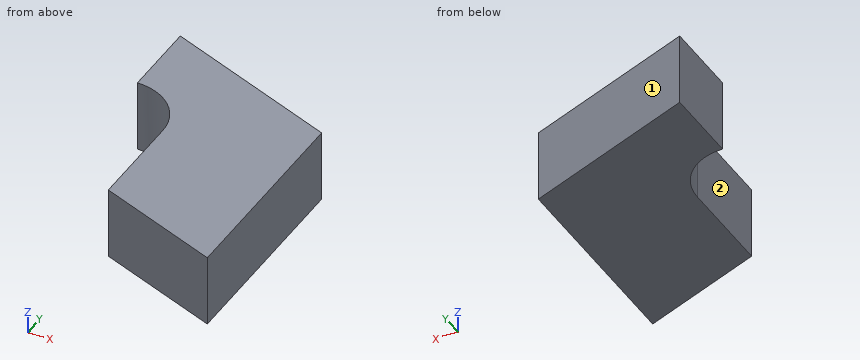
Autodesk Inventor part; units mm, degrees
ref_plane "YZ Plane" through (0, 0, 0) normal (1, 0, 0) x (0, 1, 0)
ref_plane "XZ Plane" through (0, 0, 0) normal (0, 1, 0) x (-1, 0, 0)
ref_plane "XY Plane" through (0, 0, 0) normal (0, 0, 1) x (1, 0, 0)
sketch "Sketch1" plane through (0, 0, 0) normal (0, 0, 1) x (1, 0, 0)
  line L0 (0, 0) -> (-63.5, 25.4)
  line L1 (-63.5, 25.4) -> (-63.5, 76.2)
  line L2 (-63.5, 76.2) -> (0, 76.2)
  line L3 (0, 76.2) -> (0, 0)
  line L4 (-63.5, 76.2) -> (-63.5, 101.6)
  line L5 (-63.5, 101.6) -> (0, 76.2)
  line L6 (0, 76.2) -> (0, 101.6) construction
  dimension "d0" = 76.2
  dimension "d13" = 25.4
  dimension "bottomAngle" = 68.199
  dimension "d16" = 25.4
  dimension "d17" = 68.199
  dimension "d18" = 21.801
  dimension "d19" = 63.5
extrude "Extrusion1" add sketch "Sketch1" along normal blind 25.4
sketch "Sketch2" plane through (0, 0, 25.4) normal (0, 0, 1) x (1, 0, 0)
  line L0 (-63.5, 0) -> (-44.45, 0)
  line L1 (-44.45, 0) -> (-44.45, 73.025)
  line L2 (-44.45, 73.025) -> (-63.5, 73.025)
  line L3 (-63.5, 73.025) -> (-63.5, 0)
  line L4 (-63.5, 101.6) -> (-63.5, 25.4)
  point P0 (0, 0)
  dimension "d7" = 19.05
  dimension "d8" = 73.025
extrude "Extrusion2" cut sketch "Sketch2" against normal through all
fillet "Fillet1" radius 19.05 1 edges at (-44.45, 73.025, 12.7)
sketch "Sketch3" plane through (0, 0, 25.4) normal (0, 0, 1) x (1, 0, 0)
  line L0 (-44.45, 0) -> (-3.175, 0)
  line L1 (-44.45, 53.975) -> (-44.45, 17.78)
  line L2 (0, 76.2) -> (-63.5, 101.6)
  line L3 (-3.175, 0) -> (-44.45, 16.51)
properties part number "At Angle Linear Dim"
Source: CAD feature listing. Evaluate the final solid. Frame: model axes, mm. Face numbers are marked on the shaded views. A direction names the side the tool comes from. Coordinates: 2 decimals unless noted, no trailing zeros. Loops run counter-clockwise (first coordinate to the right, second up) from the corner with the lowest first, then second, coordinate; pieces in that order, holes last. Notation, with made-up numbers: (-14, 86) -> (27, 86) arc R22 cw to (27, 108) -> close; hole circle Ø1 at (46.5, 51.5). An arc over 180 degrees is marked (long way). Answer in a Markdown table with one row per item. Add a question column.
Q1. Ray query, line 1 along X through (y, z) = (54, 22); line 2 along Y through (x, z) = (-57, 20.5). Return the intervals inside material, ascending.
Q2. Contact query for flat-ended pins moving along their axis: pin 1 Ø8 at (x, y) = (-18.5, 85) entering from +Z; pin 2 Ø8 at (x, z) = (-13, 17.5) entering from -Y; pin 3 Ø8 at (x, z) = (-54.5, 11.5) entering from -Y; pin 4 Ø1 at (y, z) = (49.5, 8.5) entering from -X. Output: stop coordinate, or through.
Q3. Section C-C on x = -4. Return the cut outline in (y, z).
Q4. Reachability of the marked faces 1 and 2 from +Z, -Z, +X, -X, +Y, -Y: full face, straight path, thin tool, end or side. Return the list, or none.
Q5. Section B-B on y = 88.5. Return the cut outline in (x, z).
Computed values:
| question | item | result |
|---|---|---|
| 1 | line 1 | x = -44.45 to 0 |
| 1 | line 2 | y = 71.88 to 99 |
| 2 | pin 1 | stops at z = 25.4 |
| 2 | pin 2 | stops at y = 3.6 |
| 2 | pin 3 | stops at y = 67.9 |
| 2 | pin 4 | stops at x = -44.45 |
| 3 | outline | (1.6, 0) -> (77.8, 0) -> (77.8, 25.4) -> (1.6, 25.4) -> close |
| 4 | face 1 | +Z, -Z, +X, +Y |
| 4 | face 2 | +Z, -Z, -X, -Y |
| 5 | outline | (-63.5, 0) -> (-30.75, 0) -> (-30.75, 25.4) -> (-63.5, 25.4) -> close |
